from build123d import *

# Parameters (mm, degrees)
SKETCH1_W           = 50.8
SKETCH1_H           = 50.8
BOSS_EXTRUDE1_DEPTH = 40.64
SKETCH2_R           = 41.91
CUT_EXTRUDE1_DEPTH  = 26.67
SKETCH3_R           = 29.21
CUT_EXTRUDE2_DEPTH  = 83.540230191
SKETCH4_R           = 2.286
CUT_EXTRUDE3_DEPTH  = 83.540230191
FILLET1_R           = 2.54
SKETCH5_R           = 3.154327094
CUT_EXTRUDE4_DEPTH  = 83.540230191


with BuildPart() as part:
    # Sketch1 → Boss-Extrude1 (new body)
    with BuildSketch(Plane.XY):
        with Locations((25.4, 25.4)):
            Rectangle(SKETCH1_W, SKETCH1_H)
    extrude(amount=BOSS_EXTRUDE1_DEPTH)

    # Sketch2 → Cut-Extrude1 (cut)
    with BuildSketch(Plane.XY.offset(40.64)):
        with Locations((6.35, 6.35)):
            Circle(SKETCH2_R)
    extrude(amount=-CUT_EXTRUDE1_DEPTH, mode=Mode.SUBTRACT)

    # Sketch3 → Cut-Extrude2 (cut, through all)
    with BuildSketch(Plane(origin=(0, 0, 0), x_dir=(-1, 0, 0), z_dir=(0, 0, -1))):
        with Locations((-6.35, 6.35)):
            Circle(SKETCH3_R)
    extrude(amount=-CUT_EXTRUDE2_DEPTH, mode=Mode.SUBTRACT)

    # Sketch4 → Cut-Extrude3 (cut, through all)
    with BuildSketch(Plane(origin=(0, 0, 0), x_dir=(-1, 0, 0), z_dir=(0, 0, -1))):
        with Locations((-6.35, 44.45)):
            Circle(SKETCH4_R)
        with Locations((-19.05, 44.45)):
            Circle(SKETCH4_R)
        with Locations((-44.45, 44.45)):
            Circle(SKETCH4_R)
        with Locations((-44.45, 31.75)):
            Circle(SKETCH4_R)
    extrude(amount=-CUT_EXTRUDE3_DEPTH, mode=Mode.SUBTRACT)

    # Fillet1
    fillet1_edges = [part.edges().sort_by_distance(p)[0] for p in [
        (0, 47.776146333, 27.305),
        (47.776146333, 0, 27.305),
        (0, 34.861429287, 6.985),
        (34.861429287, 0, 6.985),
    ]]
    fillet(fillet1_edges, radius=FILLET1_R)

    # Sketch5 → Cut-Extrude4 (cut, through all)
    with BuildSketch(Plane(origin=(0, 50.8, 0), x_dir=(1, 0, 0), z_dir=(0, 1, 0))):
        with Locations(Location((35.532091271, -28.724129848, 0), (0, 0, 270))):
            Circle(SKETCH5_R)
    extrude(amount=-CUT_EXTRUDE4_DEPTH, mode=Mode.SUBTRACT)


solid = part.part
The model under review builds one solid part; all positions refer to its coordinate system, in mm. Round coordinates to 2 decimals unless told otherwise and drop trailing zeros. Order: outer loops, then holes, each group sorted by start corner. A loop starts at its lowest first (then second) coordinate and runs counter-clockwise, first axis right, second up. Notation, with made-up numbers: (61.25, -29) - (84.25, -29) arc R14 cw to (84.25, -4) - close; hole circle Ø1 at (36.25, 36). An arc over 180 degrees is marked (long way). Use one line per item in the form item = value.
Q1. To check wall thickness, follow line 1 (Y direction, x = 19, z = 24); line 2 (Z direction, x = 28, y = 28); line 3 (X direction, y = 41, z = 28.5). State the ranges of each line that lie inside material, in increasing order.
Response values:
line_1 = 46.74 to 50.8
line_2 = 0 to 13.97
line_3 = 29.93 to 32.39, 38.68 to 50.8
Q2. Mouldability with a two-part tool opening along X and no side actions: class faces 1 (the cylindrical face through (11, 48, 27)), 2 (the cylindrical face through (46.135, 33.295, 20.036)), 3 (the flat face through (50.8, 25, 20)), 4 (the cylindrical face through (48.785, 0.801, 27.492)) as pulls with the +X half, pulls with the -X half, needs draft (parallel to the pull), parting line crosses it, or undercut.
Response values:
face_1 = undercut
face_2 = undercut
face_3 = pulls with the +X half
face_4 = pulls with the -X half
Q3. Add section D-D on x = 44.45. Give the boundary of the cut face in (y, z).
Response values:
outline = (0, 0) - (29.46, 0) - (29.46, 40.64) - (23.81, 40.64) - (23.81, 13.97) - (0, 13.97) - close; (34.04, 0) - (42.16, 0) - (42.16, 40.64) - (34.04, 40.64) - close; (46.74, 0) - (50.8, 0) - (50.8, 40.64) - (46.74, 40.64) - close
Q4. Add section B-B on x = 6.35. Give the boundary of the cut face in (y, z).
Response values:
outline = (35.56, 0) - (42.16, 0) - (42.16, 13.97) - (35.56, 13.97) - close; (46.74, 0) - (50.8, 0) - (50.8, 40.64) - (48.26, 40.64) - (48.26, 13.97) - (46.74, 13.97) - close
Q5. Clearance check with flat-ended pins moving along their axes: P1, Ø10, axis at x = 35.53, z = 28.72, coming from the -Y side; P2, Ø8, axis at x = 26, y = 36, coming from the +Z side. State where each tip first meets the part, or that it passes through.
Response values:
P1 = 30.6
P2 = 13.97
Q6. Add section C-C on z = 27. Give the boundary of the cut face in (x, y), then the cut area to 3 significant figures.
Response values:
outline = (0, 50.64) arc R2.54 ccw to (2.76, 48.11) arc R41.91 cw to (18.17, 46.56) arc R2.29 cw to (21.02, 45.61) arc R41.91 cw to (32.89, 38.79) - (32.89, 50.8) - (0, 50.8) - close; (38.17, 33.62) arc R41.91 cw to (48.11, 2.76) arc R2.54 ccw to (50.64, 0) - (50.8, 0) - (50.8, 50.8) - (38.17, 50.8) - close; hole circle Ø4.57 at (44.45, 31.75); hole circle Ø4.57 at (44.45, 44.45)
area = 517 mm^2
Q7. Add section A-A on y = 44.45. Give the boundary of the cut face in (x, z).
Response values:
outline = (0, 0) - (4.06, 0) - (4.06, 13.97) - (0, 13.97) - close; (8.64, 0) - (16.76, 0) - (16.76, 13.97) - (8.64, 13.97) - close; (21.34, 0) - (42.16, 0) - (42.16, 40.64) - (23.81, 40.64) - (23.81, 13.97) - (21.34, 13.97) - close; (46.74, 0) - (50.8, 0) - (50.8, 40.64) - (46.74, 40.64) - close; hole circle Ø6.31 at (35.53, 28.72)
